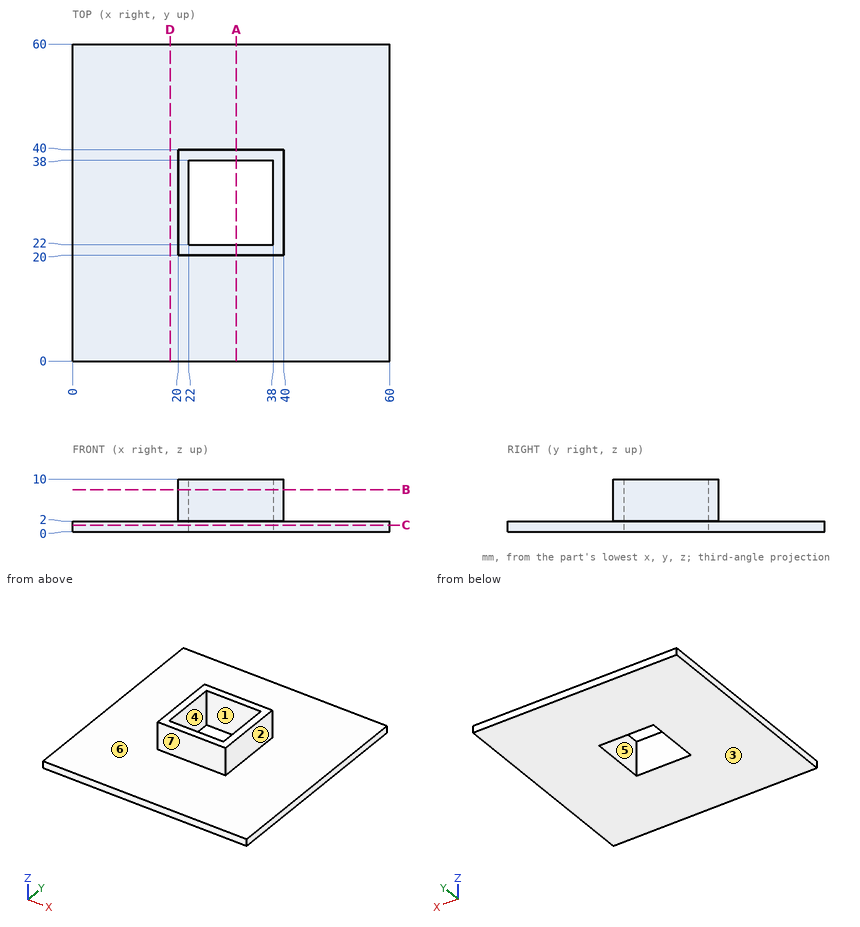
Can you work these out from the drawing? Everything is in mm from the part's minimum corner. A direction names the side the tool comes from. Give positions to 0.01 mm unless a question says otherwise; leave off trailing zeros. Loops run counter-clockwise (first coordinate to the right, second up) from the corner with the lowest first, then second, coordinate; pieces in that order, holes last. Notation, with made-up numbers: (83.25, 66) -> (98.25, 66) arc R15 cw to (98.25, 81) -> close; hole circle Ø2 at (38, -11.5). An arc over 180 degrees is marked (long way). Return JSON: item names as keys, results as strings.
Item 1: Which directions (+Z, -Z, +X, -X, +Y, -Y) give clear straight access to the entire face, cutting with the end or side of a thin tool? Please do the marked faces 1, 2 and 3.
Geometry results:
{"face 1": "+Z, -Z", "face 2": "+Z, +X, +Y, -Y", "face 3": "-Z, +X, -X, +Y, -Y"}
Item 2: If we section it at A-A on x = 31: List the corners of the cut face in (y, z) for me.
Geometry results:
{"outline": "(0, 0) -> (22, 0) -> (22, 10) -> (20, 10) -> (20, 2) -> (0, 2) -> close; (38, 0) -> (60, 0) -> (60, 2) -> (40, 2) -> (40, 10) -> (38, 10) -> close"}
Item 3: If we section it at B-B on z = 8: List the corners of the cut face in (x, y) for me, plus the area to 3 significant figures.
Geometry results:
{"outline": "(20, 20) -> (40, 20) -> (40, 40) -> (20, 40) -> close; hole (22, 22) -> (38, 22) -> (38, 38) -> (22, 38) -> close", "area": "144 mm²"}
Item 4: If we section it at C-C on z = 1.25: List the corners of the cut face in (x, y) for me.
Geometry results:
{"outline": "(0, 0) -> (60, 0) -> (60, 60) -> (0, 60) -> close; hole (22, 22) -> (38, 22) -> (38, 38) -> (22, 38) -> close"}
Item 5: We'd pull the mould along Y, two halves only. Please class the marked faces 4, 5, 6 and 7: +Y half, -Y half, draft (parallel to the pull), parting line (faces both ways), or undercut.
Geometry results:
{"face 4": "undercut", "face 5": "undercut", "face 6": "draft", "face 7": "-Y half"}
Item 6: I need wall thicknesses on L1, parallel to Y at x = 24, z = 7.75; L2, parallel to Z at x = 45, y = 13. Which ranges of each line are inside material? Lowest first, please. Write a range as from..to.
Geometry results:
{"L1": "y = 20..22, 38..40", "L2": "z = 0..2"}
Item 7: If we section it at D-D on x = 18.5: List the corners of the cut face in (y, z) for me.
Geometry results:
{"outline": "(0, 0) -> (60, 0) -> (60, 2) -> (0, 2) -> close"}
Item 8: I'm going to push flat-ended pins straight in: pin 1 (6 mm diameter, centred on x = 24, y = 15, fed in from +Z); pin 2 (3 mm diameter, centred on y = 27.5, z = 4.5, fed in from -X); pin 3 (2.5 mm diameter, centred on y = 31.5, z = 5, fed in from +X). Where does each tip first touch, or does it pass through?
Geometry results:
{"pin 1": "stops at z = 2", "pin 2": "stops at x = 20", "pin 3": "stops at x = 40"}
